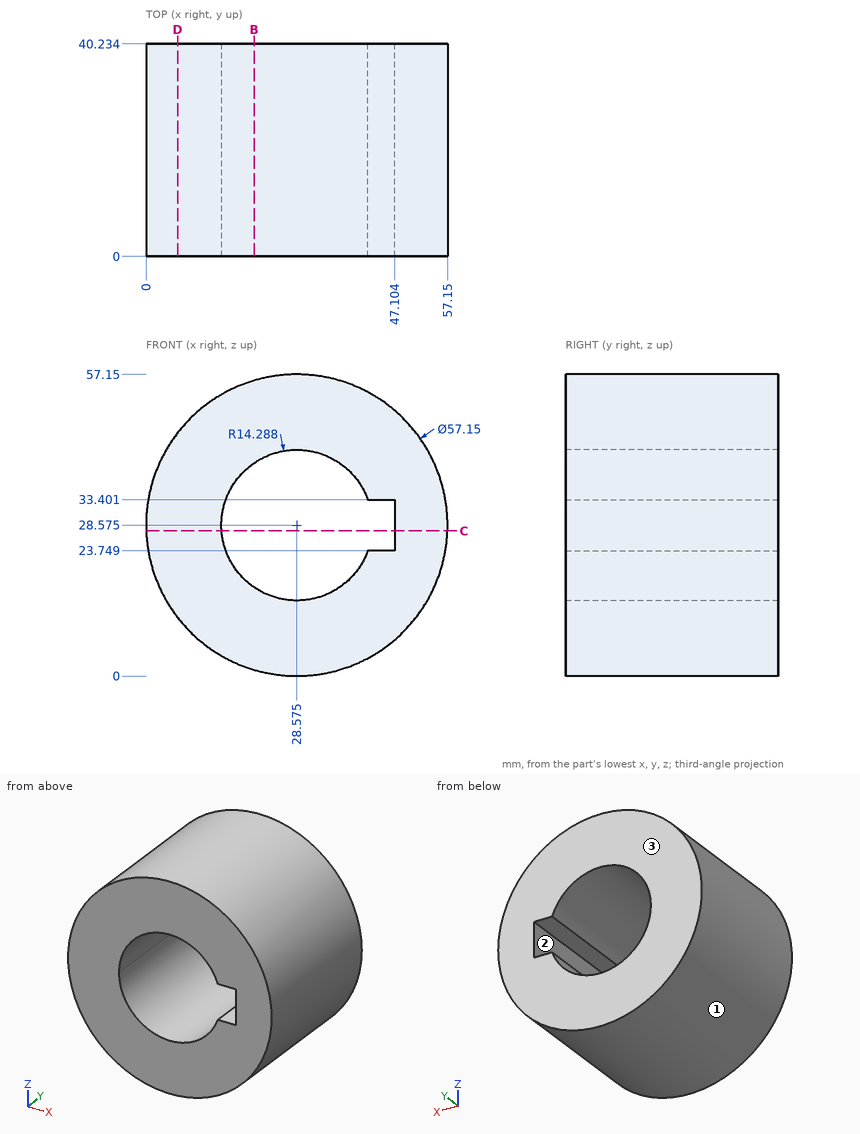
Answer from the drawing. Dimensions are ordinates in mm from the lowest x, y and z of the part. Round coordinates to 2 decimals unless told otherwise and drop trailing zeros. Order: outer loops, then holes, each group sorted by start corner. A loop starts at its lowest first (then second) coordinate and runs counter-clockwise, first axis right, second up.
1) The mould has two halves that part along X. Classify the marked faces 1, 2 and 3: released by +X, released by -X, zero draft, split by the parting line, or undercut.
2) Straight lines are drawn through the part: L1, parallel to X at y = 14.5, z = 28 (1 decimal); L2, parallel to Z at x = 24, y = 32; L3, parallel to X at y = 19, z = 30 (1 decimal). For each, find the intervals that lie inside material, in ascending order.
3) The part is cut by section D-D on x = 6. Write down the section's boundary in (y, z).
4) The part is cut by section B-B on x = 20.5. Write down the section's boundary in (y, z) (1 decimal), plus the area to 3 significant figures.
5) The part is cut by section C-C on z = 27.5. Write down the section's boundary in (x, y) (1 decimal).
6) Flat-ended cylindrical pins translate along their axes: pin 1 (8 mm diameter, centred on y = 14, z = 9, fed in from +X); pin 2 (5.5 mm diameter, centred on x = 45.5, y = 26.5, fed in from +Z) (1 decimal); pin 3 (5 mm diameter, centred on y = 24.5, z = 25.5, fed in from +X); pin 4 (7.5 mm diameter, centred on y = 27.5, z = 27, fed in from -X). Find the tip coordinate at first contact, or state that the pin passes through.
Resolved:
1. face 1: split by the parting line
1. face 2: undercut
1. face 3: zero draft
2. L1: x = 0 to 14.3, 47.1 to 57.1
2. L2: z = 0.37 to 15.04, 42.11 to 56.78
2. L3: x = 0 to 14.4, 47.1 to 57.1
3. outline: (0, 11.06) - (40.23, 11.06) - (40.23, 46.09) - (0, 46.09) - close
4. outline: (0, 1.2) - (40.2, 1.2) - (40.2, 16.8) - (0, 16.8) - close; (0, 40.4) - (40.2, 40.4) - (40.2, 56) - (0, 56) - close
4. area: 1,260 mm2
5. outline: (0, 0) - (14.3, 0) - (14.3, 40.2) - (0, 40.2) - close; (47.1, 0) - (57.1, 0) - (57.1, 40.2) - (47.1, 40.2) - close
6. pin 1: stops at x = 52.53
6. pin 2: stops at z = 53.4
6. pin 3: stops at x = 57.14
6. pin 4: stops at x = 0
